from build123d import *

# Parameters (mm, degrees)
SKETCH1_R           = 4
BOSS_EXTRUDE1_DEPTH = 35
CUT_EXTRUDE1_DEPTH  = 10
SKETCH3_R           = 2.4
CUT_EXTRUDE2_DEPTH  = 15
BOSS_EXTRUDE2_START = -7
SKETCH4_R           = 10
SKETCH4_R_2         = 4
BOSS_EXTRUDE2_DEPTH = 10


with BuildPart() as part:
    # Sketch1 → Boss-Extrude1 (new body)
    with BuildSketch(Plane(origin=(0, 0, 0), x_dir=(1, 0, 0), z_dir=(0, 1, 0))):
        with Locations(Location((0, 0, 0), (0, 0, 270))):
            Circle(SKETCH1_R)
    extrude(amount=BOSS_EXTRUDE1_DEPTH)

    # Sketch2 → Cut-Extrude1 (cut)
    with BuildSketch(Plane(origin=(0, 35, 0), x_dir=(1, 0, 0), z_dir=(0, 1, 0))):
        with BuildLine():
            Line((-1.887458609, 2), (1.887458609, 2))
            ThreePointArc((1.887458609, 2), (2.75, 0), (1.887458609, -2))
            Line((1.887458609, -2), (-1.887458609, -2))
            ThreePointArc((-1.887458609, -2), (-2.75, 0), (-1.887458609, 2))
        make_face()
    extrude(amount=-CUT_EXTRUDE1_DEPTH, mode=Mode.SUBTRACT)

    # Sketch3 → Cut-Extrude2 (cut)
    with BuildSketch(Plane(origin=(0, 0, 0), x_dir=(-1, 0, 0), z_dir=(0, -1, 0))):
        with Locations(Location((0, 0, 0), (0, 0, 90))):
            Circle(SKETCH3_R)
    extrude(amount=-CUT_EXTRUDE2_DEPTH, mode=Mode.SUBTRACT)

    # Sketch4 → Boss-Extrude2 (add)
    with BuildSketch(Plane.XZ.offset(BOSS_EXTRUDE2_START)):
        with Locations(Location((0, 0, 0), (0, 0, 270))):
            Circle(SKETCH4_R)
        with Locations(Location((0, 0, 0), (0, 0, 270))):
            Circle(SKETCH4_R_2, mode=Mode.SUBTRACT)
    extrude(amount=-BOSS_EXTRUDE2_DEPTH)


solid = part.part
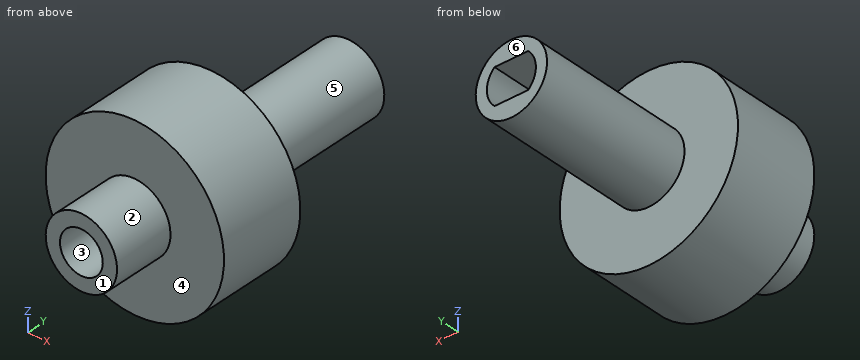
Geometry: final body of the model. Coordinates: model frame, mm. Face numbers are marked on the shaded views. A direction names the side the tool comes from. Coordinates: 2 decimals unless noted, no trailing zeros. Loops run counter-clockwise (first coordinate to the right, second up) from the corner with the lowest first, then second, coordinate; pieces in that order, holes last. Notation, with made-up numbers: M 37,33.5 L 81,33.5 A27 ccw 81,67.5 Z; hole C -7,53 d8. An arc over 180 degrees is marked long. One line per item, written item: value. Start each with the question number.
1) Cut plane A-A (z = 0). Return loops of the section in (x, y).
2) Pin query (flat end, axial travel): P1, Ø3, axis at x = 8, y = 12, coming from the +Z side; P2, Ø6, axis at x = 4.5, z = 2.5, coming from the -Y side; P3, Ø3, axis at x = -0.5, z = 0, coming from the +Y side; P4, Ø3, axis at x = -7, y = 24.5, coming from the -Z side. Return the tip coordinate at first contact, or that it passes through.
3) Cut plane B-B (y = 31.5). Return loops of the section in (x, z).
4) Reachability of the marked faces 4, 5 and 6 from +Z, -Z, +X, -X, +Y, -Y: full face, straight path, thin tool, end or side. Return the list, or none.
5) Draft query along Z for the marked faces 1, 2 and 3. Return one class per face: released by +Z, released by -Z, zero draft, split by the parting line, or undercut.
6) Cut plane C-C (x = 0). Return loops of the section in (y, z), then the cut area to 3 significant figures.
7) Material intervals for L1, parallel to X at y = 8.75, z = 0; L2, parallel to Y at x = -7, z = -0.75; L3, parallel to X at y = 4.75, z = 0, sorted ascending. Write a range as from..to.
8) Cut plane D-D (y = 6). Return loops of the section in (x, z), then the cut area to 3 significant figures.
Evaluation:
1. outline: M -10,7 L -4,7 L -4,0 L -2.4,0 L -2.4,15 L 2.4,15 L 2.4,0 L 4,0 L 4,7 L 10,7 L 10,17 L 4,17 L 4,35 L 2.75,35 L 2.75,25 L -2.75,25 L -2.75,35 L -4,35 L -4,17 L -10,17 Z
2. P1: z = 7.6
2. P2: y = 0
2. P3: y = 25
2. P4: through
3. outline: C 0,0 d8; hole M -1.89,-2 L 1.89,-2 A2.75 ccw 1.89,2 L -1.89,2 A2.75 ccw Z
4. face 4: -Y
4. face 5: +Y
4. face 6: +Z, -Z, +X, -X, +Y
5. face 1: zero draft
5. face 2: split by the parting line
5. face 3: undercut
6. outline: M 0,-4 L 7,-4 L 7,-10 L 17,-10 L 17,-4 L 35,-4 L 35,-2 L 25,-2 L 25,2 L 35,2 L 35,4 L 17,4 L 17,10 L 7,10 L 7,4 L 0,4 L 0,2.4 L 15,2.4 L 15,-2.4 L 0,-2.4 Z
6. area: 288 mm^2
7. L1: -10..-2.4, 2.4..10
7. L2: 7..17
7. L3: -4..-2.4, 2.4..4
8. outline: C 0,0 d8; hole C 0,0 d4.8
8. area: 32.2 mm^2
